from build123d import *

# Parameters (mm, degrees)
EXTRUDE_THIN1_DEPTH     = 129.2225
CUT_EXTRUDE1_DEPTH      = 1
CUT_EXTRUDE1_DEPTH_BACK = 39.1
CUT_EXTRUDE2_DEPTH      = 1
CUT_EXTRUDE2_DEPTH_BACK = 39.1


with BuildPart() as part:
    # Sketch1 → Extrude-Thin1 (new body, symmetric)
    with BuildSketch(Plane(origin=(0, 0, 0), x_dir=(0, 0, -1), z_dir=(1, 0, 0))):
        with BuildLine():
            Line((-15.875, 19.05), (15.875, 19.05))
            ThreePointArc((15.875, 19.05), (18.12006403, 18.12006403), (19.05, 15.875))
            Line((19.05, 15.875), (19.05, -15.875))
            ThreePointArc((19.05, -15.875), (18.12006403, -18.12006403), (15.875, -19.05))
            Line((15.875, -19.05), (-15.875, -19.05))
            ThreePointArc((-15.875, -19.05), (-18.12006403, -18.12006403), (-19.05, -15.875))
            Line((-19.05, -15.875), (-19.05, 15.875))
            ThreePointArc((-19.05, 15.875), (-18.12006403, 18.12006403), (-15.875, 19.05))
        make_face()
        with BuildLine():
            Line((-15.875, 16.51), (15.875, 16.51))
            ThreePointArc((15.875, 16.51), (16.324012806, 16.324012806), (16.51, 15.875))
            Line((16.51, 15.875), (16.51, -15.875))
            ThreePointArc((16.51, -15.875), (16.324012806, -16.324012806), (15.875, -16.51))
            Line((15.875, -16.51), (-15.875, -16.51))
            ThreePointArc((-15.875, -16.51), (-16.324012806, -16.324012806), (-16.51, -15.875))
            Line((-16.51, -15.875), (-16.51, 15.875))
            ThreePointArc((-16.51, 15.875), (-16.324012806, 16.324012806), (-15.875, 16.51))
        make_face(mode=Mode.SUBTRACT)
    extrude(amount=EXTRUDE_THIN1_DEPTH, both=True)

    # Sketch2 → Cut-Extrude1 (cut, two sides)
    with BuildSketch(Plane.XY.offset(19.05)) as cut_extrude1_sk:
        Polygon((-395.460759114, -480.188191704), (-129.2225, -19.05), (-107.225454744, 19.05), (159.01280437, 480.188191704), (-763.263579039, 1012.664709933), (-1317.737142523, 52.288326524), align=None)
    extrude(amount=CUT_EXTRUDE1_DEPTH, mode=Mode.SUBTRACT)
    extrude(cut_extrude1_sk.sketch, amount=-CUT_EXTRUDE1_DEPTH_BACK, mode=Mode.SUBTRACT)

    # Sketch3 → Cut-Extrude2 (cut, two sides)
    with BuildSketch(Plane.XY.offset(19.05)) as cut_extrude2_sk:
        Polygon((395.460759114, -480.188191704), (129.2225, -19.05), (107.225454744, 19.05), (-159.01280437, 480.188191704), (763.263579039, 1012.664709933), (1317.737142523, 52.288326524), align=None)
    extrude(amount=CUT_EXTRUDE2_DEPTH, mode=Mode.SUBTRACT)
    extrude(cut_extrude2_sk.sketch, amount=-CUT_EXTRUDE2_DEPTH_BACK, mode=Mode.SUBTRACT)


solid = part.part
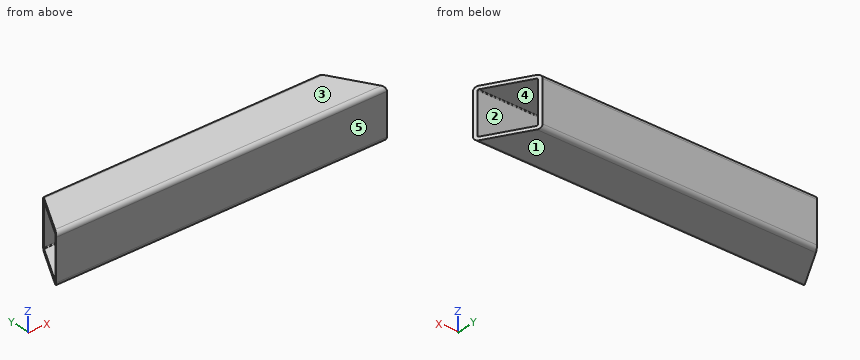
Source: CAD feature listing. Evaluate the final solid. Frame: model axes, mm. Face numbers are marked on the shaded views. A direction names the side the tool comes from. Round coordinates to 2 decimals unless told otherwise and drop trailing zeros. Write each loop counter-clockwise with the first axis right and the second up, starting at its lowest first coordinate (ties: lowest second). Pieces come first, ordered by that corner, then holes. Notation, with made-up numbers: (37.5, -9.75) - (60.5, -9.75) arc R11 cw to (60.5, 7.25) - close; hole circle Ø4 at (-4.75, 23). An arc over 180 degrees is marked (long way). Use CSV: the item, a comma, the result in double quotes. Start each with the question number.
(1) Material intervals for probe 1 along Y at (x, z) = (-27.5, -3); probe 2 along Y at (x, z) = (110.5, 2), sorted ascending. Write a range as [from, to].
(2) Cut plane B-B, the plane y = -4.5. Return loops of the section in (x, z).
(3) First-contact query: pin 1 Ø3 at (y, z) = (-12.5, 14.5) entering from -X. Flat tip, straight axial feed; report the tip coordinate or a pass-through.
(4) Cut plane A-A, the plane z = 8. Return loops of the section in (x, y), and give its area (3 significant figures).
(5) Cut plane C-C, the plane x = -76.5. Return loops of the section in (y, z) (3 decimals).
(6) Mould query, pull axis Z, two halves, no side actions, for the marked faces 1, 2 and 3. Classes: pulls with the +Z half, pulls with the -Z half, needs draft (parallel to the pull), parting line crosses it, or undercut.
(7) Set-up query: the marked faces 4 and 5. Return all of +Z, -Z, +X, -X, +Y, -Y with unobstructed straight access to the full face (end or side cutting, diameter ignored); none if empty.
Geometry says:
1,probe 1,"[-19.05, -16.51], [16.51, 19.05]"
1,probe 2,"[-19.05, -16.51]"
2,outline,"(-120.82, -19.05) - (120.82, -19.05) - (120.82, -16.51) - (-120.82, -16.51) - close; (-120.82, 16.51) - (120.82, 16.51) - (120.82, 19.05) - (-120.82, 19.05) - close"
3,pin 1,"through"
4,outline,"(-129.22, -19.05) - (129.22, -19.05) - (127.76, -16.51) - (-127.76, -16.51) - close; (-108.69, 16.51) - (108.69, 16.51) - (107.23, 19.05) - (-107.23, 19.05) - close"
4,area,"1,200 mm²"
5,outline,"(-19.05, -15.875) arc R3.175 ccw to (-15.875, -19.05) - (15.875, -19.05) arc R3.175 ccw to (19.05, -15.875) - (19.05, 15.875) arc R3.175 ccw to (15.875, 19.05) - (-15.875, 19.05) arc R3.175 ccw to (-19.05, 15.875) - close; hole (-16.51, -15.875) arc R0.635 ccw to (-15.875, -16.51) - (15.875, -16.51) arc R0.635 ccw to (16.51, -15.875) - (16.51, 15.875) arc R0.635 ccw to (15.875, 16.51) - (-15.875, 16.51) arc R0.635 ccw to (-16.51, 15.875) - close"
6,face 1,"pulls with the -Z half"
6,face 2,"undercut"
6,face 3,"pulls with the +Z half"
7,face 4,"+X, -X"
7,face 5,"+Z, -Z, +X, -X, -Y"
